Source: CAD feature listing. Evaluate the final solid. Frame: model axes, mm. Face numbers are marked on the shaded views. A direction names the side the tool comes from. Coordinates: 2 decimals unless noted, no trailing zeros. Loops run counter-clockwise (first coordinate to the right, second up) from the corner with the lowest first, then second, coordinate; pieces in that order, holes last.
Autodesk Inventor part; units mm, degrees
ref_plane "YZ Plane" through (0, 0, 0) normal (1, 0, 0) x (0, 1, 0)
ref_plane "XZ Plane" through (0, 0, 0) normal (0, 1, 0) x (-1, 0, 0)
ref_plane "XY Plane" through (0, 0, 0) normal (0, 0, 1) x (1, 0, 0)
sketch "Sketch1" plane through (0, 0, 0) normal (1, 0, 0) x (0, 1, 0)
  line L0 (52.4, 0) -> (4, 0)
  line L1 (0, -4) -> (0, -52.4)
  line L2 (4, -56.4) -> (52.4, -56.4)
  line L3 (56.4, -52.4) -> (56.4, -4)
  line L4 (51.77, -4.63) -> (4.63, -4.63) construction
  line L5 (4.63, -4.63) -> (4.63, -51.77) construction
  line L6 (4.63, -51.77) -> (51.77, -51.77) construction
  line L7 (51.77, -51.77) -> (51.77, -4.63) construction
  circle A0 centre (51.77, -4.63) radius 2.5
  circle A1 centre (51.77, -51.77) radius 2.5
  circle A2 centre (4.63, -4.63) radius 2.5
  circle A3 centre (4.63, -51.77) radius 2.5
  arc A4 (56.4, -4) -> (52.4, 0) centre (52.4, -4) ccw
  arc A5 (52.4, -56.4) -> (56.4, -52.4) centre (52.4, -52.4) ccw
  arc A6 (0, -52.4) -> (4, -56.4) centre (4, -52.4) ccw
  arc A7 (4, 0) -> (0, -4) centre (4, -4) ccw
  point P0 (0, 0)
  point P1 (56.4, 0)
  point P2 (0, 0)
  point P3 (56.4, -56.4)
  point P4 (56.4, -28.2)
  point P5 (51.77, -28.2)
  point P6 (28.2, -51.77)
  point P7 (28.2, -56.4)
  dimension "d0" = 56.4
  dimension "d1" = 47.14
  dimension "d2" = 5
  dimension "d3" = 4
  dimension "d4" = 4
  dimension "d5" = 4
  dimension "d6" = 4
extrude "Extrusion1" add sketch "Sketch1" along normal blind 76
sketch "Sketch2" plane through (0, 0, 0) normal (-1, 0, 0) x (0, 0, 1)
  circle A0 centre (-28.2, 28.2) radius 19.05
  line L0 (-52.4, 56.4) -> (-4, 56.4)
  line L1 (-56.4, 4) -> (-56.4, 52.4)
  point P0 (0, 0)
  point P1 (-28.2, 56.4)
  point P2 (-56.4, 28.2)
  dimension "d9" = 38.1
extrude "Extrusion2" add sketch "Sketch2" along normal blind 1.6
sketch "Sketch3" plane through (-1.6, 28.2, -28.2) normal (-1, 0, 0) x (0, 0, 1)
  circle A0 centre (0, 0) radius 3.175
  circle A1 centre (0, 0) radius 19.05 construction
  point P0 (28.2, -28.2)
  dimension "d12" = 6.35
extrude "Extrusion3" add sketch "Sketch3" along normal blind 24
properties part number "Nema23"
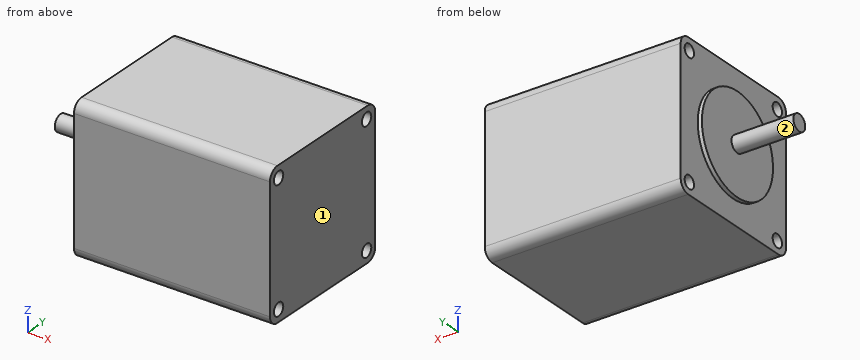
Q1. Reachability of the marked faces 1 and 2 from +Z, -Z, +X, -X, +Y, -Y: full face, straight path, thin tool, end or side. Return the list, or none.
Q2. Material intervals for line 1 along Y through (x, z) = (49.5, -4.5); line 2 along Z through (x, y) = (54, 51.77); line 3 along Y through (x, z) = (40, -4), sorted ascending.
Q3. Section query D-D on x = -19. Return the cut outline in (y, z) (3 decimals), then the cut area to 3 significant figures.
Q4. Section query A-A on x = 65. Return the cut outline in (y, z), then the cut area to 3 significant figures.
Q5. Section query B-B on z = -28.2. Return the cut outline in (x, y) (3 decimals).
Q6. Section query C-C on y = 28.2. Return the cut outline in (x, z) (3 decimals), then the cut area to 3 significant figures.
Q7. First-contact query: pin 1 Ø4 at (x, z) = (54, -48.5) entering from -Y; pin 2 Ø6.5 at (y, z) = (4.63, -51.77) entering from -X; pin 3 Ø4.5 at (y, z) = (51.77, -51.77) entering from -X; pin 4 Ø5 at (y, z) = (46, -20.5) entering from -X. Flat tips, straight axial feed; report the tip coordinate or a pass-through.
Resolved:
1. face 1: +Z, -Z, +X, +Y, -Y
1. face 2: -X
2. line 1: y = 0 to 2.13, 7.13 to 49.27, 54.27 to 56.4
2. line 2: z = -56.4 to -54.27, -49.27 to -7.13, -2.13 to 0
2. line 3: y = 0 to 2.21, 7.05 to 49.35, 54.19 to 56.4
3. outline: circle Ø6.35 at (28.2, -28.2)
3. area: 31.7 mm2
4. outline: (0, -52.4) arc R4 ccw to (4, -56.4) - (52.4, -56.4) arc R4 ccw to (56.4, -52.4) - (56.4, -4) arc R4 ccw to (52.4, 0) - (4, 0) arc R4 ccw to (0, -4) - close; hole circle Ø5 at (4.63, -51.77); hole circle Ø5 at (4.63, -4.63); hole circle Ø5 at (51.77, -51.77); hole circle Ø5 at (51.77, -4.63)
4. area: 3,090 mm2
5. outline: (-25.6, 25.025) - (-1.6, 25.025) - (-1.6, 9.15) - (0, 9.15) - (0, 0) - (76, 0) - (76, 56.4) - (0, 56.4) - (0, 47.25) - (-1.6, 47.25) - (-1.6, 31.375) - (-25.6, 31.375) - close
6. outline: (-25.6, -31.375) - (-1.6, -31.375) - (-1.6, -47.25) - (0, -47.25) - (0, -56.4) - (76, -56.4) - (76, 0) - (0, 0) - (0, -9.15) - (-1.6, -9.15) - (-1.6, -25.025) - (-25.6, -25.025) - close
6. area: 4,500 mm2
7. pin 1: stops at y = 0
7. pin 2: stops at x = 0
7. pin 3: passes through
7. pin 4: stops at x = -1.6
